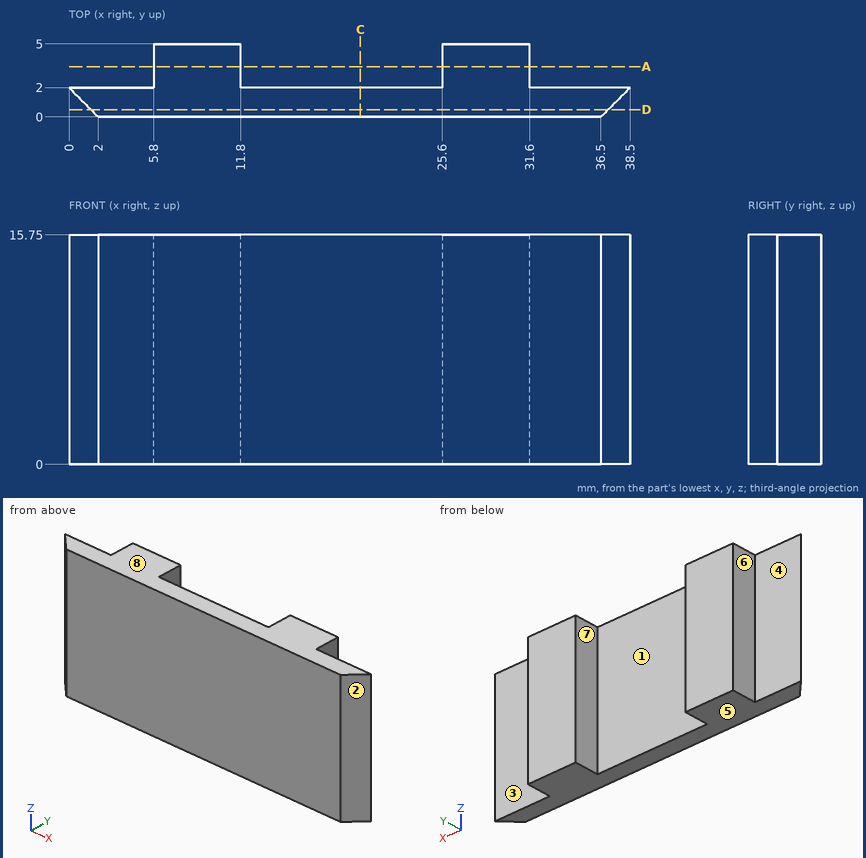
Design review of the part shown in the three views and the two pictorial views. Dimensions are in mm from the part's minimum x, y and z. A direction names the side the tool comes from. Round coordinates to 2 decimals unless told otherwise and drop trailing zeros. Order: outer loops, then holes, each group sorted by start corner. A loop starts at its lowest first (then second) coordinate and runs counter-clockwise, first axis right, second up. Notation, with made-up numbers: (-5, 19.5) - (25, 19.5) arc R27 ccw to (25, 55.5) - close; hole circle Ø3 at (68, 84.25). An arc over 180 degrees is marked (long way). One line per question, with ' | ' between items.
Item 1: Machinability: for the marked faces 1, 2, 3, 4 and 5, which of the approach directions +Z, -Z, +X, -X, +Y, -Y give a long, thin tool a straight path to every point of the face, cutting with its end or side? Answer none if there is none.
Checks:
face 1: +Z, -Z, +Y | face 2: +Z, -Z, +X, -Y | face 3: +Z, -Z, +X, +Y | face 4: +Z, -Z, -X, +Y | face 5: -Z, +X, -X, +Y, -Y
Item 2: Draft analysis for pull direction X (two halves, no side actions). For the marked faces 6, 7 and 8, state which applies: +X half, -X half, draft (parallel to the pull), parting line (faces both ways), or undercut.
Checks:
face 6: -X half | face 7: undercut | face 8: draft
Item 3: Wall thickness on line 1 (X direction, y = 2.95, z = 13.75); line 2 (Y direction, x = 5, z = 11.25); line 3 (X direction, y = 0.9, z = 14.25): over which ranges is each line inside the solid? List them lowest first. Write a range as [from, to].
Checks:
line 1: [5.8, 11.8], [25.6, 31.6] | line 2: [0, 2] | line 3: [1.1, 37.4]
Item 4: Take a section at D-D, the plane y = 0.5. Write out the cut boundary in (x, z), then the cut area to 3 significant figures.
Checks:
outline: (1.5, 0) - (37, 0) - (37, 15.75) - (1.5, 15.75) - close | area: 559 mm²
Item 5: Take a section at C-C, the plane x = 20. Write out the cut boundary in (y, z).
Checks:
outline: (0, 0) - (2, 0) - (2, 15.75) - (0, 15.75) - close
Item 6: For P1, Ø1.5, axis at y = 3.5, z = 9.5, coming from the -X side; P2, Ø2.5, axis at y = 3.5, z = 8.5, coming from the +X side; P3, Ø1, axis at y = 0.5, z = 6.5, coming from the -X side, all flat-tipped, find the tip position at first contact; note any pin that passes through.
Checks:
P1: x = 5.8 | P2: x = 31.6 | P3: x = 1
Item 7: Take a section at A-A, the plane y = 3.45. Write out the cut boundary in (x, z).
Checks:
outline: (5.8, 0) - (11.8, 0) - (11.8, 15.75) - (5.8, 15.75) - close; (25.6, 0) - (31.6, 0) - (31.6, 15.75) - (25.6, 15.75) - close
